Input: part model. Units: mm. Frame: model coordinates. Face numbers are marked on the shaded views. Coordinates: 2 decimals unless noted, no trailing zeros. Order: outer loops, then holes, each group sorted by start corner. A loop starts at its lowest first (then second) coordinate and runs counter-clockwise, first axis right, second up. Notation, with made-up numbers: M -2,28 L 27,28 A19 cw 27,46 Z; hole C 61,61 d2. An arc over 180 degrees is marked long. One line per item, written item: value.
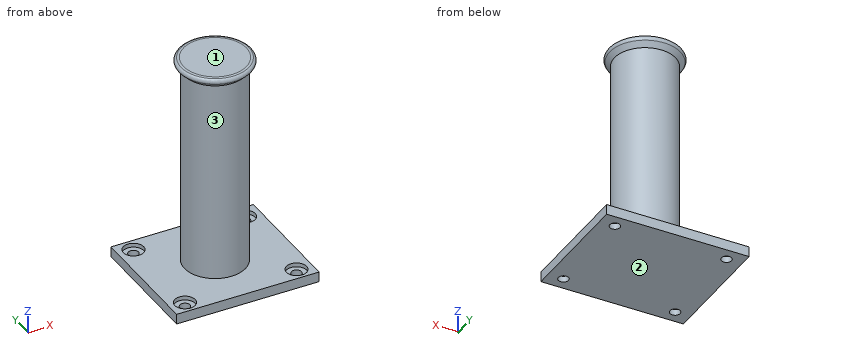
```python
from build123d import *

# Parameters (mm, degrees)
F0_W           = 70
F0_H           = 60
F0_R           = 15
F1_DEPTH       = 5
F2_DEPTH       = 105
F3_R           = 18.75
F3_R_2         = 15
F4_DEPTH       = 5
F5_SIZE        = 3.74999
F7_R           = 1.5
F9_D           = 5
F9_DEPTH       = 5
F9_CBORE_D     = 10
F9_CBORE_DEPTH = 2
F9_TIP         = 1.5021515476


# Not quite as in the source:
# - a fillet or chamfer that OpenCascade refuses, or shapes differently, is made with other operations: its cross-section is extruded or revolved along the edge and cut away or added
# - a fillet or chamfer is up to 0.001 mm smaller than in the source, because OpenCascade refuses the exact size


with BuildPart() as f1:
    # F0 (on Top) → F1 (new body)
    with BuildSketch(Plane.XY):
        Rectangle(F0_W, F0_H)
        Circle(F0_R, mode=Mode.SUBTRACT)
    extrude(amount=F1_DEPTH)

    # F0 (on Top) → F2 (join)
    with BuildSketch(Plane.XY):
        Circle(F0_R)
    extrude(amount=F2_DEPTH)

    # F3 (on face) → F4 (join)
    with BuildSketch(Plane.XY.offset(105)):
        Circle(F3_R)
        Circle(F3_R_2, mode=Mode.SUBTRACT)
        Circle(F3_R_2)
    extrude(amount=F4_DEPTH)

    # F5 (size 3.75 in the source; OpenCascade refuses exactly that, so slightly less here)
    f5_edges = [f1.edges().sort_by_distance(p)[0] for p in [
        (-18.75, 0, 105),
    ]]
    chamfer(f5_edges, length=F5_SIZE)

    # F6: fillet of radius 5 on 1 edges, made by hand

    # F6_s1 → F6_t2 (revolve, cut)
    with BuildSketch(Plane.XZ):
        with BuildLine():
            ThreePointArc((18.75, 108.74999), (17.2105735463, 109.6770690609), (15.4427995223, 110))
            Line((15.4427995223, 110), (18.75, 110))
            Line((18.75, 110), (18.75, 108.74999))
        make_face()
    revolve(axis=Axis((0, 0, 110), (0, 0, 1)), mode=Mode.SUBTRACT)

    # F7
    f7_edges = [f1.edges().sort_by_distance(p)[0] for p in [
        (-18.75, 0, 108.74999),
    ]]
    fillet(f7_edges, radius=F7_R)

    # F9
    with Locations(Plane.XY.offset(5)):
        with Locations((-27.4074339763, 23.4920862654), (-27.4074339763, -23.4920862654), (27.4074339763, -23.4920862654), (27.4074339763, 23.4920862654)):
            CounterBoreHole(F9_D / 2, F9_CBORE_D / 2, F9_CBORE_DEPTH, depth=F9_DEPTH)
            with Locations((0, 0, -(F9_DEPTH + F9_TIP / 2))):  # 118° drill point
                Cone(0, F9_D / 2, F9_TIP, mode=Mode.SUBTRACT)


solid = f1.part
```
(1) Draft query along Z for the marked faces 1, 2 and 3. Return one class per face: released by +Z, released by -Z, zero draft, split by the parting line, or undercut.
Data:
face 1: released by +Z
face 2: released by -Z
face 3: undercut
(2) Ray query, line 1 (Z direction, x = -19.5, y = 3); line 2 (Z direction, x = 30.5, y = -20.5); line 3 (Z direction, x = 16.5, y = 2.5). Return the intervals inside material, ascending. Write a range as from..to.
Data:
line 1: z = 0..5
line 2: z = 0..3
line 3: z = 0..5, 106.69..109.84
(3) Cut plane A-A on z = 52.5. Output: boundary loops of the cut face in (x, y).
Data:
outline: C 0,0 d30
(4) Cut plane B-B on x = -19.5. Output: boundary loops of the cut face in (y, z), plus the area to 3 significant figures.
Data:
outline: M -30,0 L 30,0 L 30,5 L -30,5 Z
area: 300 mm2
(5) First-contact query: pin 1 (3 mm diameter, centred on x = -30, y = 26, fed in from +Z); pin 2 (6 mm diameter, centred on y = 4, z = 23.5, fed in from +X); pin 3 (8 mm diameter, centred on y = -15.5, z = 59.5, fed in from +X); pin 4 (4 mm diameter, centred on x = 27.41, y = -23.49, fed in from +Z). Flat tips, straight axial feed; report the tip coordinate or a pass-through.
Data:
pin 1: stops at z = 5
pin 2: stops at x = 14.97
pin 3: stops at x = 9.63
pin 4: passes through
